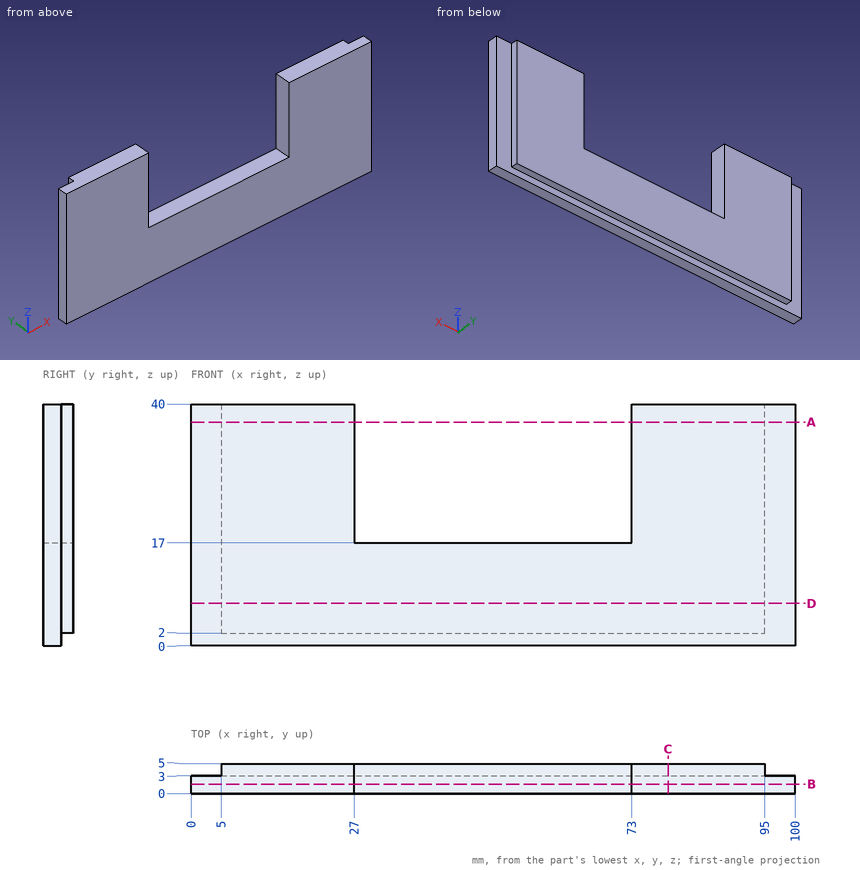
Here's the drawing with two shaded views (mm, measured from the low corner). I have some questions. Coordinates: 2 decimals unless noted, no trailing zeros. Loops run counter-clockwise (first coordinate to the right, second up) from the corner with the lowest first, then second, coordinate; pieces in that order, holes last. Notation, with made-up numbers: (21, 23.5) -> (46, 23.5) arc R31 ccw to (46, 52.5) -> close; hole circle Ø7 at (-13.5, 12.5). An arc over 180 degrees is marked (long way). Use one line per item in the form item = value. Start each with the question number.
(1) If we section it at D-D (z = 7): Please give me the cut outline in (x, y), then the cut area to 3 significant figures.
(2) Please list where these lines run through material, in increasing order: line 1 along X through (y, z) = (2.35, 25); line 2 along Z through (x, y) = (35, 3.1); line 3 along Z through (x, y) = (94.5, 4.5).
(3) If we section it at B-B (y = 1.6): Please give me the cut outline in (x, z).
(4) If we section it at C-C (x = 79): Please give me the cut outline in (y, z).
(5) If we section it at A-A (z = 37): Please give me the cut outline in (x, y).
(6) Will these pins go through, and if not, where does the flat tip stop? pin 1 (1.6 mm diameter, centred on y = 4, z = 26, fed in from +X); pin 2 (0.6 mm diameter, centred on x = 61, y = 4, fed in from -Z); pin 3 (2.5 mm diameter, centred on x = 40.5, y = 3.5, fed in from +Z).
Verdict:
q1.outline = (0, 0) -> (100, 0) -> (100, 3) -> (95, 3) -> (95, 5) -> (5, 5) -> (5, 3) -> (0, 3) -> close
q1.area = 480 mm²
q2.line_1 = 0 to 27, 73 to 100
q2.line_2 = 2 to 17
q2.line_3 = 2 to 40
q3.outline = (0, 0) -> (100, 0) -> (100, 40) -> (73, 40) -> (73, 17) -> (27, 17) -> (27, 40) -> (0, 40) -> close
q4.outline = (0, 0) -> (3, 0) -> (3, 2) -> (5, 2) -> (5, 40) -> (0, 40) -> close
q5.outline = (0, 0) -> (27, 0) -> (27, 5) -> (5, 5) -> (5, 3) -> (0, 3) -> close; (73, 0) -> (100, 0) -> (100, 3) -> (95, 3) -> (95, 5) -> (73, 5) -> close
q6.pin_1 = 95
q6.pin_2 = 2
q6.pin_3 = 17
